from build123d import *
from build123d.topology import SkipClean

# Parameters (mm, degrees)
BOSS_EXTRUDE1_DEPTH      = 20
SKETCH3_W                = 78
SKETCH3_H                = 10
CUT_EXTRUDE1_DEPTH       = 108.29864864
SKETCH5_W                = 20
SKETCH5_H                = 10
CUT_EXTRUDE2_DEPTH       = 88.321245983
BOSS_EXTRUDE3_DEPTH      = 72
SKETCH10_R               = 18
CUT_EXTRUDE4_DEPTH       = 113.058020686
SKETCH11_R               = 6
CUT_EXTRUDE5_DEPTH       = 88.321245983
SKETCH14_R               = 18
SKETCH14_R_2             = 9
BOSS_EXTRUDE4_DEPTH      = 72
SKETCH19_R               = 18
CUT_EXTRUDE6_DEPTH       = 9
BOSS_EXTRUDE5_DEPTH      = 9
BOSS_EXTRUDE5_DEPTH_BACK = 63
CUT_EXTRUDE8_DEPTH       = 42.619271
BOSS_EXTRUDE6_DEPTH      = 5
BOSS_EXTRUDE7_DEPTH      = 5


with BuildPart() as part:
    # Sketch1 → Boss-Extrude1 (new body)
    with BuildSketch(Plane(origin=(0, 0, 0), x_dir=(1, 0, 0), z_dir=(0, 1, 0))):
        with BuildLine():
            Line((-26, -77), (26, -77))
            ThreePointArc((26, -77), (33.071067812, -74.071067812), (36, -67))
            Line((36, -67), (36, 77))
            Line((36, 77), (-36, 77))
            Line((-36, 77), (-36, -67))
            ThreePointArc((-36, -67), (-33.071067812, -74.071067812), (-26, -77))
        make_face()
    extrude(amount=BOSS_EXTRUDE1_DEPTH)

    # Sketch3 → Cut-Extrude1 (cut, through all)
    with BuildSketch(Plane.ZY.offset(36)):
        with Locations((38, 5)):
            Rectangle(SKETCH3_W, SKETCH3_H)
    extrude(amount=-CUT_EXTRUDE1_DEPTH, mode=Mode.SUBTRACT)

    # Sketch5 → Cut-Extrude2 (cut, through all)
    with BuildSketch(Plane(origin=(0, 20, 0), x_dir=(1, 0, 0), z_dir=(0, 1, 0))):
        with Locations((0, -72)):
            Rectangle(SKETCH5_W, SKETCH5_H)
    extrude(amount=-CUT_EXTRUDE2_DEPTH, mode=Mode.SUBTRACT)

    # Sketch9 → Boss-Extrude3 (add, through all)
    with BuildSketch(Plane.ZY.offset(36)):
        with BuildLine():
            ThreePointArc((52.419027344, 21.741935484), (26.054797228, 37.984041733), (0.846606339, 20))
            Line((0.846606339, 20), (12.033370453, 20))
            ThreePointArc((12.033370453, 20), (27, 28), (41.966629547, 20))
            Line((41.966629547, 20), (53.153393661, 20))
            Line((53.153393661, 20), (55.142494559, 20))
            ThreePointArc((55.142494559, 20), (53.526046841, 20.472729382), (52.419027344, 21.741935484))
        make_face()
        with BuildLine():
            ThreePointArc((41.966629547, 20), (44.22497216, 15.22497216), (45, 10))
            Line((45, 10), (55, 10))
            ThreePointArc((55, 10), (54.534478591, 15.08453427), (53.153393661, 20))
            Line((53.153393661, 20), (41.966629547, 20))
        make_face()
        with BuildLine():
            ThreePointArc((0.846606339, 20), (-0.534478591, 15.08453427), (-1, 10))
            Line((-1, 10), (9, 10))
            ThreePointArc((9, 10), (9.77502784, 15.22497216), (12.033370453, 20))
            Line((12.033370453, 20), (0.846606339, 20))
        make_face()
    extrude(amount=-BOSS_EXTRUDE3_DEPTH)

    # Sketch10 → Cut-Extrude4 (cut, through all)
    with SkipClean():  # the faces are left unmerged after this step: merging them gives an invalid solid
        with BuildSketch(Plane.ZY.offset(36)):
            with Locations((27, 10)):
                Circle(SKETCH10_R)
        extrude(amount=-CUT_EXTRUDE4_DEPTH, mode=Mode.SUBTRACT)

    # Sketch11 → Cut-Extrude5 (cut, through all)
    with SkipClean():  # the faces are left unmerged after this step: merging them gives an invalid solid
        with BuildSketch(Plane(origin=(0, 20, 0), x_dir=(1, 0, 0), z_dir=(0, 1, 0))):
            with Locations(Location((-18, 19.367183159, 0), (0, 0, 270))):
                Circle(SKETCH11_R)
        cut_extrude5 = extrude(amount=-CUT_EXTRUDE5_DEPTH, mode=Mode.SUBTRACT)

    # Mirror1: Cut-Extrude5 across plane
    with SkipClean():  # the faces are left unmerged after this step: merging them gives an invalid solid
        add(cut_extrude5.mirror(Plane(origin=(0, 0, 0), x_dir=(0, 0, 1), z_dir=(1, 0, 0))), mode=Mode.SUBTRACT)



with BuildPart() as body_2:
    # Sketch14 → Boss-Extrude4 (new, through all)
    with BuildSketch(Plane.ZY.offset(36)):
        with Locations((-37.91461026, 82)):
            Circle(SKETCH14_R)
        with Locations((-37.91461026, 82)):
            Circle(SKETCH14_R_2, mode=Mode.SUBTRACT)
    extrude(amount=-BOSS_EXTRUDE4_DEPTH)

    # Sketch19 → Cut-Extrude6 (cut)
    with BuildSketch(Plane.ZY.offset(36)):
        with Locations((-37.91461026, 82)):
            Circle(SKETCH19_R)
    cut_extrude6 = extrude(amount=-CUT_EXTRUDE6_DEPTH, mode=Mode.SUBTRACT)

    # Mirror2: Cut-Extrude6 across plane
    add(cut_extrude6.mirror(Plane(origin=(0, 0, 0), x_dir=(0, 0, 1), z_dir=(1, 0, 0))), mode=Mode.SUBTRACT)

    # Sketch21 → Boss-Extrude5 (add, two sides: drawn at the far end of the back side and taken through both)
    with BuildSketch(Plane.ZY.offset(27).offset(-BOSS_EXTRUDE5_DEPTH_BACK)):
        with BuildLine():
            Line((-32.209949075, 19.927892902), (-43.619271445, 19.927892902))
            Line((-43.619271445, 19.927892902), (-43.619271445, 64.927892902))
            ThreePointArc((-43.619271445, 64.927892902), (-37.91461026, 64), (-32.209949075, 64.927892902))
            Line((-32.209949075, 64.927892902), (-32.209949075, 19.927892902))
        make_face()
    extrude(amount=BOSS_EXTRUDE5_DEPTH + BOSS_EXTRUDE5_DEPTH_BACK)

    # Sketch24 → Cut-Extrude8 (cut)
    with BuildSketch(Plane(origin=(0, 0, -43.619271445), x_dir=(-1, 0, 0), z_dir=(0, 0, -1))):
        Polygon((-27, 64.927892902), (-27, 54.927892902), (-36, 20), (-36, 64.927892902), align=None)
        Polygon((27, 64.927892902), (27, 54.927892902), (36, 20), (36, 64.927892902), align=None)
    extrude(amount=-CUT_EXTRUDE8_DEPTH, mode=Mode.SUBTRACT)


with BuildPart() as part_1:
    with SkipClean():  # the faces are left unmerged after this step: merging them gives an invalid solid
        add(part.part)

        add(body_2.part)  # Boss-Extrude6 merges body 2
        # Sketch30 → Boss-Extrude6 (add, symmetric)
        with BuildSketch(Plane(origin=(0, 0, 0), x_dir=(0, 0, -1), z_dir=(1, 0, 0))):
            with BuildLine():
                Line((-45.750774329, 30.794433439), (25.860541049, 95.367850068))
                ThreePointArc((25.860541049, 95.367850068), (20.293859016, 78.324523758), (32.209949075, 64.927892902))
                Line((32.209949075, 64.927892902), (32.209949075, 20))
                Line((32.209949075, 20), (-0.846606339, 20))
                ThreePointArc((-0.846606339, 20), (-20.455564076, 37.224444135), (-45.750774329, 30.794433439))
            make_face()
        extrude(amount=BOSS_EXTRUDE6_DEPTH, both=True)

    # Sketch31 → Boss-Extrude7 (add, symmetric)
    with SkipClean():  # the faces are left unmerged after this step: merging them gives an invalid solid
        with BuildSketch(Plane(origin=(0, 0, 0), x_dir=(0, 0, -1), z_dir=(1, 0, 0))):
            with BuildLine():
                Line((43.619271445, 64.927892902), (43.619271445, 20))
                Line((43.619271445, 20), (77, 20))
                Line((77, 20), (55.032581189, 87.565525247))
                ThreePointArc((55.032581189, 87.565525247), (53.987373983, 73.896527516), (43.619271445, 64.927892902))
            make_face()
        extrude(amount=BOSS_EXTRUDE7_DEPTH, both=True)


solid = part_1.part
Geometry: final body of the model. Coordinates: model frame, mm. A direction names the side the tool comes from. Round coordinates to 2 decimals unless told otherwise and drop trailing zeros. Order: outer loops, then holes, each group sorted by start corner. A loop starts at its lowest first (then second) coordinate and runs counter-clockwise, first axis right, second up. Notation, with made-up numbers: (6.5, 66.25) -> (46.5, 66.25) arc R17 cw to (46.5, 85.25) -> close; hole circle Ø5 at (22, 4). An arc over 180 degrees is marked (long way). Put each result on its own line as item: value. Start each with the question number.
Q1. Reachability of faces 5 (the cylindrical face through (-9, 38, 27)), 6 (the flat face through (-1, 10, 4)), 7 (the flat face through (20, 20, -61)) from +Z, -Z, +X, -X, +Y, -Y: full face, straight path, thin tool, end or side. Return the list, or none.
Q2. Section B-B on x = -2.5. Return the cut outline in (y, z), and give its area (3 significant figures).
Q3. Section A-A on x = -18. Return the cut outline in (y, z).
Q4. First-contact query: pin 1 (16 mm diameter, centred on x = -11, z = 68.5, fed in from -Y); pin 2 (9.5 mm diameter, centred on x = -20.5, z = -63.5, fed in from +Y); pin 3 (4 mm diameter, centred on x = 0, z = 50, fed in from +Y). Flat tips, straight axial feed; report the tip coordinate or a pass-through.
Q5. Section C-C on y = 82. Return the cut outline in (x, z), and give its area (3 significant figures).
Q6. Line query: probe 1 along Z at (x, y) = (18, 15.25); probe 2 along Y at (x, z) = (-23, -31); probe 3 along Z at (x, y) = (-17, 81.5). Output: solid intervals per line, ascending.
Q7. Section D-D on z = -18. Return the cut outline in (x, y), and give its area (3 significant figures).
Q8. Pull-direction query (X, two-part tool) for faces 1 (the cylindrical face through (-13.945, 10.14, -23.789)), 2 (the flat face through (27, 72.8, -38.2)), 3 (the flat face through (-10, 15, 72)), 4 (the flat face through (1, 10, -77)); classes: +X half, -X half, draft (parallel to the pull), parting line (faces both ways), or undercut.
Ans:
1. face 5: +Y
1. face 6: +Z, +X, -X, -Y
1. face 7: -Z, +X
2. outline: (0, -77) -> (20, -77) -> (87.57, -55.03) arc R18 ccw to (95.37, -25.86) -> (30.79, 45.75) arc R28 ccw to (21.74, 52.42) arc R3 cw to (20, 55.14) -> (20, 67) -> (10, 67) -> (10, 45) arc R18 cw to (10, 9) -> (10, -1) -> (0, -1) -> close; hole circle Ø18 at (82, -37.91)
2. area: 7,570 mm2
3. outline: (0, -77) -> (20, -77) -> (20, -43.62) -> (64.93, -43.62) arc R18 ccw (long way) to (64.93, -32.21) -> (20, -32.21) -> (20, -25.37) -> (0, -25.37) -> close; (0, -13.37) -> (20, -13.37) -> (20, 0.85) arc R28 ccw to (21.74, 52.42) arc R3 cw to (20, 55.14) -> (20, 77) -> (10, 77) -> (10, 45) arc R18 cw to (10, 9) -> (10, -1) -> (0, -1) -> close; hole circle Ø18 at (82, -37.91)
4. pin 1: stops at y = 10
4. pin 2: stops at y = 20
4. pin 3: stops at y = 28.52
5. outline: (-27, -55.91) -> (-5, -55.91) -> (-5, -56.84) -> (5, -56.84) -> (5, -55.91) -> (27, -55.91) -> (27, -46.91) -> (-27, -46.91) -> close; (-27, -28.91) -> (27, -28.91) -> (27, -19.91) -> (5, -19.91) -> (5, -11.04) -> (-5, -11.04) -> (-5, -19.91) -> (-27, -19.91) -> close
5. area: 1,070 mm2
6. probe 1: z = -77 to -25.37, -13.37 to 9.78, 44.22 to 77
6. probe 2: y = 0 to 20, 65.38 to 76.24, 87.76 to 98.62
6. probe 3: z = -55.91 to -46.9, -28.93 to -19.92
7. outline: (-36, 0) -> (-23.84, 0) -> (-23.84, 20) -> (-36, 20) -> close; (-12.16, 0) -> (12.16, 0) -> (12.16, 20) -> (5, 20) -> (5, 88.28) -> (-5, 88.28) -> (-5, 20) -> (-12.16, 20) -> close; (23.84, 0) -> (36, 0) -> (36, 20) -> (23.84, 20) -> close
7. area: 1,660 mm2
8. face 1: undercut
8. face 2: +X half
8. face 3: undercut
8. face 4: draft
